Here's how the part is built. I have some questions about the finished solid (model axes, mm). A direction names the side the tool comes from. Give positions to 0.01 mm unless a question says otherwise; leave off trailing zeros. Order: outer loops, then holes, each group sorted by start corner. A loop starts at its lowest first (then second) coordinate and runs counter-clockwise, first axis right, second up. Notation, with made-up numbers: M 29.25,83 L 56.25,83 A21 cw 56.25,103 Z; hole C 56.25,88 d1. An arc over 180 degrees is marked long. Use one line per item in the form item = value.
from build123d import *

# Parameters (mm, degrees)
SKETCH_1_W      = 2.54
SKETCH_1_H      = 17.78
EXTRUDE_1_DEPTH = 11
SKETCH_2_W      = 40
SKETCH_2_H      = 27.78
SKETCH_2_R      = 1.7500127
SKETCH_2_R_2    = 1.75
EXTRUDE_2_DEPTH = 1.6


with BuildPart() as part:
    # 草图1 → 凸台-拉伸1 (new body)
    with BuildSketch(Plane.XY):
        with Locations((-9.398018796, 46.482082804)):
            Rectangle(SKETCH_1_W, SKETCH_1_H)
    extrude(amount=EXTRUDE_1_DEPTH)

    # 草图2 → 凸台-拉伸2 (add)
    with BuildSketch(Plane.XY.offset(11)):
        with Locations((-27.728018796, 48.482082804)):
            Rectangle(SKETCH_2_W, SKETCH_2_H)
        with Locations((-10.439420879, 59.35991872)):
            Circle(SKETCH_2_R, mode=Mode.SUBTRACT)
        with Locations((-43.840487681, 59.35991872)):
            Circle(SKETCH_2_R_2, mode=Mode.SUBTRACT)
        with Locations((-43.840487681, 38.023876048)):
            Circle(SKETCH_2_R_2, mode=Mode.SUBTRACT)
    extrude(amount=EXTRUDE_2_DEPTH)


solid = part.part
Q1. I want a section at C-C on y = 39.25. Write out the boundary of the cut face in (x, z), then the cut area to 3 significant figures.
Found:
outline = M -47.73,11 L -45.09,11 L -45.09,12.6 L -47.73,12.6 Z; M -42.59,11 L -10.67,11 L -10.67,0 L -8.13,0 L -8.13,11 L -7.73,11 L -7.73,12.6 L -42.59,12.6 Z
area = 87.9 mm²
Q2. I want a section at D-D on z = 10.25. Write out the boundary of the cut face in (x, y).
Found:
outline = M -10.67,37.59 L -8.13,37.59 L -8.13,55.37 L -10.67,55.37 Z
Q3. I need wall thicknesses on L1, parallel to X at y = 59, z = 11.25; L2, parallel to Z at x = -35.5, y = 44.25; L3, parallel to X at y = 49.25, z = 7. Which ranges of each line are inside material? Lowest first, please.
Found:
L1 = -47.73 to -45.55, -42.13 to -12.15, -8.73 to -7.73
L2 = 11 to 12.6
L3 = -10.67 to -8.13
Q4. On a 3-axis mill with a long thin cutter (end or side, diameter ignored), from which of +Z, -Z, +X, -X, +Y, -Y can I reach the whole of each face in a straight line? I mean faces 5 (the face through (-9, 37.592, 5)), 6 (the face through (-8.128, 46, 5)), 7 (the face through (-9, 55.372, 5)), 8 (the face through (-10.668, 46, 5)). Say none if no direction works.
Found:
face_5 = -Z, +X, -X, -Y
face_6 = -Z, +X, +Y, -Y
face_7 = -Z, +X, -X, +Y
face_8 = -Z, -X, +Y, -Y
Q5. Thinking about a two-plate mould opening in X: for faces 1 (the face through (-10.82, 57.65, 11.79)), 2 (the face through (-7.728, 48, 12)), 3 (the face through (-42.9, 39.5, 11.8)), 4 (the face through (-28, 34.592, 12)), which applies, +X half, -X half, draft (parallel to the pull), parting line (faces both ways), or undercut?
Found:
face_1 = undercut
face_2 = +X half
face_3 = undercut
face_4 = draft
Q6. I'm going to push flat-ended pins straight in: pin 1 Ø1.5 at (x, y) = (-37.5, 39) entering from -Z; pin 2 Ø1.3 at (x, z) = (-10, 8) entering from +Y; pin 3 Ø2 at (y, z) = (38.5, 4.5) entering from -X. Where does each tip first touch, or does it pass through?
Found:
pin_1 = 11
pin_2 = 55.37
pin_3 = -10.67
Q7. I want a section at A-A on y = 49.5. Write out the boundary of the cut face in (x, z), then the cut area to 3 significant figures.
Found:
outline = M -47.73,11 L -10.67,11 L -10.67,0 L -8.13,0 L -8.13,11 L -7.73,11 L -7.73,12.6 L -47.73,12.6 Z
area = 91.9 mm²
Q8. I want a section at B-B on x = -43. Write out the boundary of the cut face in (y, z), then the cut area to 3 significant figures.
Found:
outline = M 34.59,11 L 36.49,11 L 36.49,12.6 L 34.59,12.6 Z; M 39.56,11 L 57.82,11 L 57.82,12.6 L 39.56,12.6 Z; M 60.89,11 L 62.37,11 L 62.37,12.6 L 60.89,12.6 Z
area = 34.6 mm²
